Autodesk Inventor part; units mm, degrees
ref_plane "YZ Plane" through (0, 0, 0) normal (1, 0, 0) x (0, 1, 0)
ref_plane "XZ Plane" through (0, 0, 0) normal (0, 1, 0) x (-1, 0, 0)
ref_plane "XY Plane" through (0, 0, 0) normal (0, 0, 1) x (1, 0, 0)
sketch "Sketch1" plane through (0, 0, 0) normal (0, 1, 0) x (-1, 0, 0)
  line L0 (0, 0) -> (78, 0)
  line L1 (78, 0) -> (78, -70)
  line L2 (78, -70) -> (0, -70)
  line L3 (0, -70) -> (0, 0)
  line L4 (0, 0) -> (10, 0)
  line L5 (10, 0) -> (10, -70)
  line L6 (10, -70) -> (0, -70)
  line L7 (0, -70) -> (0, 0)
  line L8 (10, 0) -> (10, -10)
  line L9 (10, -10) -> (10, -34.9935)
  line L10 (10, -34.9935) -> (10, -59.987)
  line L11 (78, -70) -> (68, -70)
  line L12 (68, -70) -> (68, 0)
  line L13 (68, 0) -> (78, 0)
  line L14 (78, 0) -> (78, -70)
  line L15 (68, -70) -> (68, -60.4)
  line L16 (68, -60.4) -> (68, -9.6)
  circle A0 centre (68, -60.4) radius 6.25
  circle A1 centre (68, -9.6) radius 6.25
  line L17 (0, 0) -> (18.2, 0)
  line L18 (18.2, 0) -> (18.2, -70)
  line L19 (18.2, -70) -> (0, -70)
  line L20 (0, -70) -> (0, 0)
  line L21 (18.2, -70) -> (28.2, -70)
  line L22 (28.2, -70) -> (28.2, 0)
  line L23 (28.2, 0) -> (18.2, 0)
  line L24 (18.2, 0) -> (18.2, -70)
  dimension "d0" = 78
  dimension "d1" = 70
  dimension "d2" = 10
  dimension "d3" = 10
  dimension "d4" = 24.9935
  dimension "d5" = 24.9935
  dimension "d27" = 10
  dimension "d28" = 9.6
  dimension "d29" = 50.8
  dimension "d30" = 12.5
  dimension "d31" = 12.5
  dimension "d49" = 18.2
  dimension "d50" = 10
extrude "Extrusion1" add sketch "Sketch1" along normal blind 15
sketch "Sketch2" plane through (0, 15, 0) normal (0, 1, 0) x (1, 0, 0)
  line L0 (-78, 70) -> (-78, 0)
  line L1 (-78, 0) -> (0, 0)
  line L2 (-78, 70) -> (-68, 70)
  line L3 (-68, 70) -> (-68, 0)
  line L4 (-68, 0) -> (-78, 0)
  line L5 (-78, 0) -> (-78, 70)
  line L6 (-68, 70) -> (-68, 60.4)
  line L7 (-68, 60.4) -> (-68, 9.6)
  line L8 (0, 70) -> (-78, 70)
  line L9 (-68, 0) -> (-28.2, 0)
  line L10 (-28.2, 0) -> (-28.2, 70)
  line L11 (-28.2, 70) -> (-68, 70)
  line L12 (-68, 70) -> (-68, 0)
  line L13 (-28.2, 70) -> (-18.2, 70)
  line L14 (-18.2, 70) -> (-18.2, 0)
  line L15 (-18.2, 0) -> (-28.2, 0)
  line L16 (-28.2, 0) -> (-28.2, 70)
  line L17 (-28.2, 0) -> (-23.2, 0)
  line L18 (-23.2, 0) -> (-23.2, 70)
  line L19 (-23.2, 70) -> (-28.2, 70)
  line L20 (-28.2, 70) -> (-28.2, 0)
  line L21 (-23.2, 0) -> (-23.2, 8)
  line L22 (-23.2, 8) -> (-23.2, 26)
  line L23 (-23.2, 26) -> (-23.2, 44)
  line L24 (-23.2, 44) -> (-23.2, 62)
  line L25 (-23.2, 62) -> (-23.2, 70)
  point P0 (-28.2, 0)
  dimension "d15" = 10
  dimension "d16" = 9.6
  dimension "d17" = 50.8
  dimension "d25" = 39.8
  dimension "d26" = 10
  dimension "d36" = 5
  dimension "d37" = 8
  dimension "d38" = 18
  dimension "d39" = 18
  dimension "d40" = 18
  dimension "d41" = 8
extrude "Extrusion2" add sketch "Sketch1" against normal blind 12 contours A1 L12 | L12 A1 | A0 L12 | L12 A0
hole "Hole1" at (-10, 0, -10) at (-10, 0, -34.9935) at (-10, 0, -59.987) direction (0, 1, 0) diameter 6.2 end through all counterbore diameter 11 counterbore depth 8
hole "Hole2" at (-68, 15, -60.4) at (-68, 15, -9.6) direction (0, -1, 0) diameter 6.5 end through all counterbore diameter 11.113 counterbore depth 8
hole "Hole3" at (-23.2, 15, -62) at (-23.2, 15, -44) at (-23.2, 15, -26) at (-23.2, 15, -8) direction (0, -1, 0) diameter 4.2 end through all counterbore diameter 8 counterbore depth 6
extrude "Extrusion4" cut sketch "Sketch1" along normal blind 4 contours L0 L22 L2 L18
properties part number "CameraAdapter_part1"
Geometry check sheet. Reference: the model listing, model coordinates, mm. A direction names the side the tool comes from. Give positions to 0.01 mm unless a question says otherwise; leave off trailing zeros. Order: outer loops, then holes, each group sorted by start corner. A loop starts at its lowest first (then second) coordinate and runs counter-clockwise, first axis right, second up.
1. Section check D-D, the plane y = 10.5. Give the number of separate pieces and of enclosed holes in the cut face, and give its area (3 significant figures).
2. Access from +Z, -Z, +X, -X, +Y, -Y to the whole of each face (thin tool, end or side, straight path). Record for faces 1 (the face through (-21, 9, -6)), 2 (the face through (-8.114, 11.549, -32.533)), 3 (the face through (-23, 4, -35)), 4 (the face through (-7.89, 4.06, -15.08)), 5 (the face through (-40, 7, -70)).
3. Section check C-C, the plane y = 1.75. Enter the section's corners in (x, z), and give its area (3 significant figures).
4. Gauge pin test, flat ends, axial feed: pin 1 Ø9 at (x, z) = (-67, -9.5) entering from +Y; pin 2 Ø4 at (x, z) = (-24, -44.5) entering from +Y; pin 3 Ø9 at (x, z) = (-25, -63.5) entering from +Y; pin 4 Ø12 at (x, z) = (-9, -61.5) entering from -Y. Record the tip position at first contact, or that the pin passes through.
5. Section check A-A, the plane z = -26. Enter the section's corners in (x, y), and give its area (3 significant figures).
6. Thickness scan on L1, parallel to Z at x = -23.2, y = 10.35; L2, parallel to Z at x = -10, y = 12.75; L3, parallel to Z at x = -10, y = 5. Record the ranges inside material, lowest first.
7. Section check B-B, the plane x = -10. Enter the section's corners in (y, z).
8. Release check for a two-part mould opening along Z. For faces 6 (the face through (-7.6, 8, -37.4)), 7 (the face through (-38, 7, 0)), 8 (the face through (0, 7, -35)) record: pulls with the +Z half, pulls with the -Z half, needs draft (parallel to the pull), parting line crosses it, or undercut.
Values follow:
1. separate pieces: 1
1. enclosed holes: 9
1. area: 4,970 mm2
2. face 1: +Y
2. face 2: +Y, -Y
2. face 3: +Z, -Z, -Y
2. face 4: -Y
2. face 5: -Z, +X, -X, +Y, -Y
3. outline: (-78, -70) - (-28.2, -70) - (-28.2, 0) - (-78, 0) - close; (-18.2, -70) - (0, -70) - (0, 0) - (-18.2, 0) - close; hole circle Ø6.5 at (-68, -60.4); hole circle Ø6.5 at (-68, -9.6); hole circle Ø11 at (-10, -59.99); hole circle Ø11 at (-10, -34.99); hole circle Ø11 at (-10, -10)
3. area: 4,410 mm2
4. pin 1: stops at y = 7
4. pin 2: stops at y = 9
4. pin 3: stops at y = 15
4. pin 4: stops at y = 0
5. outline: (-78, 0) - (-28.2, 0) - (-28.2, 4) - (-25.3, 4) - (-25.3, 9) - (-27.2, 9) - (-27.2, 15) - (-78, 15) - close; (-21.1, 4) - (-18.2, 4) - (-18.2, 0) - (0, 0) - (0, 15) - (-19.2, 15) - (-19.2, 9) - (-21.1, 9) - close
5. area: 1,060 mm2
6. L1: z = -70 to -66, -58 to -48, -40 to -30, -22 to -12, -4 to 0
6. L2: z = -70 to -63.09, -56.89 to -38.09, -31.89 to -13.1, -6.9 to 0
6. L3: z = -70 to -65.49, -54.49 to -40.49, -29.49 to -15.5, -4.5 to 0
7. outline: (0, -70) - (15, -70) - (15, -63.09) - (8, -63.09) - (8, -65.49) - (0, -65.49) - close; (0, -54.49) - (8, -54.49) - (8, -56.89) - (15, -56.89) - (15, -38.09) - (8, -38.09) - (8, -40.49) - (0, -40.49) - close; (0, -29.49) - (8, -29.49) - (8, -31.89) - (15, -31.89) - (15, -13.1) - (8, -13.1) - (8, -15.5) - (0, -15.5) - close; (0, -4.5) - (8, -4.5) - (8, -6.9) - (15, -6.9) - (15, 0) - (0, 0) - close
8. face 6: undercut
8. face 7: pulls with the +Z half
8. face 8: needs draft
